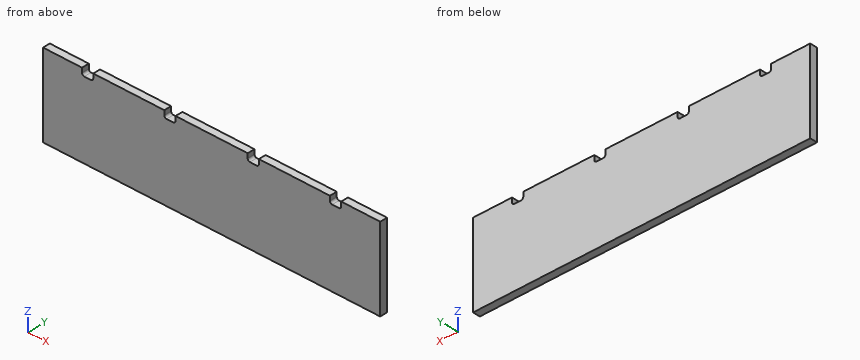
Autodesk Inventor part; units mm, degrees
ref_plane "YZ Plane" through (0, 0, 0) normal (1, 0, 0) x (0, 1, 0)
ref_plane "XZ Plane" through (0, 0, 0) normal (0, 1, 0) x (-1, 0, 0)
ref_plane "XY Plane" through (0, 0, 0) normal (0, 0, 1) x (1, 0, 0)
sketch "Sketch1" plane through (0, 0, 0) normal (0, 1, 0) x (-1, 0, 0)
  line L0 (0, 0) -> (-300, 0)
  line L1 (-300, 0) -> (-300, -74.151)
  line L2 (-300, -74.151) -> (0, -74.151)
  line L3 (0, -74.151) -> (0, 0)
  dimension "d0" = 300
  dimension "d1" = 74.151
extrude "Extrusion1" add sketch "Sketch1" along normal blind 6.5
sketch "Sketch2" plane through (0, 6.5, 0) normal (0, 1, 0) x (1, 0, 0)
  line L0 (0, 0) -> (300, 0)
  line L1 (300, 74.151) -> (0, 74.151)
  line L2 (150, 74.151) -> (150, 0) construction
  line L3 (34.711, 0) -> (44.711, 0)
  line L4 (44.711, 0) -> (44.711, 4)
  line L5 (42.711, 6) -> (36.711, 6)
  line L6 (34.711, 4) -> (34.711, 0)
  line L7 (107.911, 0) -> (117.911, 0)
  line L8 (117.911, 0) -> (117.911, 4)
  line L9 (115.911, 6) -> (109.911, 6)
  line L10 (107.911, 4) -> (107.911, 0)
  arc A0 (36.711, 6) -> (34.711, 4) centre (36.711, 4) ccw
  arc A1 (44.711, 4) -> (42.711, 6) centre (42.711, 4) ccw
  arc A2 (109.911, 6) -> (107.911, 4) centre (109.911, 4) ccw
  arc A3 (117.911, 4) -> (115.911, 6) centre (115.911, 4) ccw
  line L11 (265.289, 0) -> (255.289, 0)
  line L12 (255.289, 0) -> (255.289, 4)
  line L13 (257.289, 6) -> (263.289, 6)
  line L14 (265.289, 4) -> (265.289, 0)
  line L15 (192.089, 0) -> (182.089, 0)
  line L16 (182.089, 0) -> (182.089, 4)
  line L17 (184.089, 6) -> (190.089, 6)
  line L18 (192.089, 4) -> (192.089, 0)
  arc A4 (265.289, 4) -> (263.289, 6) centre (263.289, 4) ccw
  arc A5 (257.289, 6) -> (255.289, 4) centre (257.289, 4) ccw
  arc A6 (192.089, 4) -> (190.089, 6) centre (190.089, 4) ccw
  arc A7 (184.089, 6) -> (182.089, 4) centre (184.089, 4) ccw
  point P0 (39.711, 6)
  point P1 (112.911, 6)
  point P2 (260.289, 6)
  point P3 (187.089, 6)
  dimension "d10" = 2
  dimension "d11" = 73.2
  dimension "d12" = 37.089
  dimension "d13" = 10
  dimension "d14" = 10
  dimension "d15" = 6
extrude "Extrusion2" cut sketch "Sketch2" against normal through all
equation "\"d13\" = d14"
properties part number "front_panel_bottom"
Design review of the part built by this model. Coordinates are the model's own, in mm. Coordinates: 2 decimals unless noted, no trailing zeros. Order: outer loops, then holes, each group sorted by start corner. A loop starts at its lowest first (then second) coordinate and runs counter-clockwise, first axis right, second up. Notation, with made-up numbers: (8.25, 67.5) - (28.25, 67.5) arc R6 cw to (28.25, 72.5) - close; hole circle Ø3 at (66.5, 52). An arc over 180 degrees is marked (long way). One line per question, with ' | ' between items.
Q1. Clearance check with flat-ended pins moving along their axes: pin 1 Ø1.8 at (x, y) = (259.5, 2) entering from +Z; pin 2 Ø1.5 at (x, z) = (144, -9) entering from -Y. State where each tip first meets the part, or that it passes through.
Answer key:
pin 1: stops at z = -6 | pin 2: stops at y = 0
Q2. To check wall thickness, follow line 1 along Z through (x, y) = (258.5, 5.5). State the ranges of the line that lie inside material, in increasing order.
Answer key:
line 1: z = -74.15 to -6
Q3. Consider section A-A, the plane x = 113. Give the boundary of the cut face in (y, z), then the cut area to 3 significant figures.
Answer key:
outline: (0, -74.15) - (6.5, -74.15) - (6.5, -6) - (0, -6) - close | area: 443 mm2
